Build history of the part. All positions in model axes, mm. Face numbers are marked on the shaded views. A direction names the side the tool comes from. Give positions to 0.01 mm unless a question says otherwise; leave off trailing zeros. Loops run counter-clockwise (first coordinate to the right, second up) from the corner with the lowest first, then second, coordinate; pieces in that order, holes last. Notation, with made-up numbers: (47, -2.5) - (60, -2.5) arc R24 ccw to (60, 34.5) - close; hole circle Ø3 at (-24, 25.5). An arc over 180 degrees is marked (long way). Return JSON: item names as keys, results as strings. Group by question number.
1) 3-axis set-ups, long thin cutter, end or side, ignore diameter. For the marked faces 5, 6 and 7: which of +Z, -Z, +X, -X, +Y, -Y reach the whole face in a straight line?
2) Slice it at B-B (z = 1.75). List the corners of the cut face in (x, y) (3 decimals), and give its area (3 significant figures).
3) Drill centre lines: probe 1 along Z at (x, y) = (10.5, 0.1) (1 decimal); probe 2 along X at (y, z) = (1.2, -9.5); probe 3 along X at (y, z) = (-0.05, -6). Where is each one in solid material? Low to high. Write a range as from..to.
4) Drop flat-ended pins along their axis: pin 1 (1 mm diameter, centred on x = 7.5, y = 0, fed in from +Z) (3 decimals); pin 2 (1 mm diameter, centred on x = -7, y = 1, fed in from -Z); pin 3 (1.5 mm diameter, centred on y = 0.5, z = 8.5, fed in from +X); pin 4 (3 mm diameter, centred on x = -5.5, z = -6, fed in from +Y) (3 decimals). Give the stop position or say it passes through.
5) Slice it at A-A (x = -0.5). List the corners of the cut face in (y, z) (3 decimals).
6) Mould opens along Z. For the marked faces 1, 2, 3 and 4 say: released by +Z, released by -Z, zero draft, split by the parting line, or undercut.
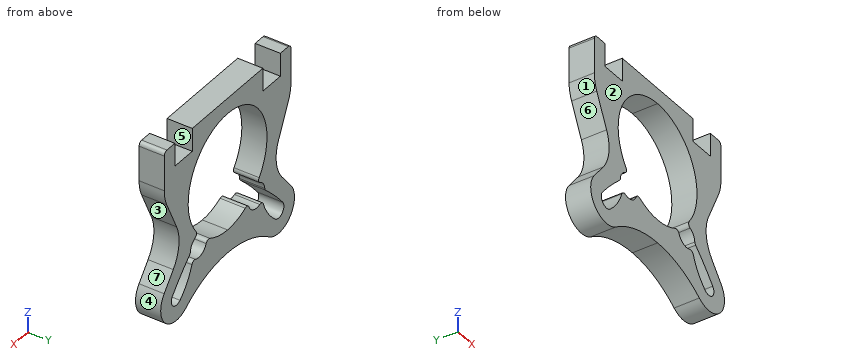
```python
from build123d import *
from build123d import SkipClean  # not in build123d's __all__

# Parameters (mm, degrees)
F2_DEPTH = 1.625
F3_R     = 0.5
F4_R     = 5


with BuildPart() as f2:
    # F1 (on Front) → F2 (new body, symmetric)
    with BuildSketch(Plane.XZ):
        with BuildLine():
            ThreePointArc((0, -6.875), (-2.0724417463, -6.5551971906), (-3.9520768911, -5.6255411515))
            ThreePointArc((-3.9520768911, -5.6255411515), (-4.8570002775, -7.1160909953), (-6.5757097792, -6.8217054979))
            ThreePointArc((-6.5757097792, -6.8217054979), (-7.4894639741, -8.9857797177), (-9.0066893746, -10.7791539234))
            ThreePointArc((-9.0066893746, -10.7791539234), (-10.3561219729, -10.7473840389), (-10.4445927673, -9.400479966))
            ThreePointArc((-10.4445927673, -9.400479966), (-8.8177667586, -7.5260240462), (-7.0479231089, -5.7859661986))
            ThreePointArc((-7.0479231089, -5.7859661986), (-6.6159518229, -4.6300438958), (-5.4766665535, -4.1559293139))
            ThreePointArc((-5.4766665535, -4.1559293139), (-6.837727437, 3.9011833784), (0, 8.375))
            Line((0, 8.375), (0, 10.375))
            Line((0, 10.375), (-6.6871520114, 10.375))
            Line((-6.6871520114, 10.375), (-6.6871520114, 7.375))
            Line((-6.6871520114, 7.375), (-9.9871520114, 7.375))
            Line((-9.9871520114, 7.375), (-9.9871520114, 10.375))
            Line((-9.9871520114, 10.375), (-11.9871520114, 10.375))
            Line((-11.9871520114, 10.375), (-11.9871520114, 4.2244328171))
            Line((-11.9871520114, 4.2244328171), (-8.5746230978, -3.0885299193))
            ThreePointArc((-8.5746230978, -3.0885299193), (-8.458137965, -3.3292198832), (-8.3348983214, -3.5665222959))
            Line((-8.3348983214, -3.5665222959), (-12.0057025921, -8.1503055323))
            ThreePointArc((-12.0057025921, -8.1503055323), (-11.8324993376, -12.098674705), (-7.8959026306, -12.4491384793))
            ThreePointArc((-7.8959026306, -12.4491384793), (-4.1524531082, -10.534781214), (0, -9.875))
            Line((0, -9.875), (0, -6.875))
        make_face()
    extrude(amount=F2_DEPTH, both=True)

    # F3
    f3_edges = [f2.edges().sort_by_distance(p)[0] for p in [
        (-3.952077, 0, -5.625541),
        (-7.047923, 0, -5.785966),
        (-11.987152, 0, 10.375),
        (-5.476667, 0, -4.155929),
        (-6.57571, 0, -6.821705),
    ]]
    fillet(f3_edges, radius=F3_R)

    # F4
    f4_edges = [f2.edges().sort_by_distance(p)[0] for p in [
        (-8.334898, 0, -3.566522),
        (-11.987152, 0, 4.224433),
    ]]
    fillet(f4_edges, radius=F4_R)

    # F5: F2 across plane


with BuildPart() as f2_1:
    add(f2.part, clean=False)
    with SkipClean():  # cleaning this boolean's faces spoils the solid; the shape is the same uncleaned
        add(f2.part.mirror(Plane.YZ), clean=False)


solid = f2_1.part
```
Results:
{
 "1": {"face 5": "+Z, +Y, -Y", "face 6": "-X, +Y, -Y", "face 7": "+X, +Y, -Y"},
 "2": {"outline": "(-10.832, -1.625) - (-7.415, -1.625) - (-7.415, 1.625) - (-10.832, 1.625) - close; (7.415, -1.625) - (10.832, -1.625) - (10.832, 1.625) - (7.415, 1.625) - close", "area": "22.2 mm2"},
 "3": {"probe 1": "-12.9..-10.6, -9.5..-6.3, 1..10.4", "probe 2": "-12.62..-10.51, -7.83..7.83, 10.51..12.62", "probe 3": "-10.28..-7.28, -3.82..-3.36, 3.36..3.82, 7.28..10.28"},
 "4": {"pin 1": "z = 7.375", "pin 2": "z = -12.17", "pin 3": "x = 11.99", "pin 4": "y = 1.625"},
 "5": {"outline": "(-1.625, -9.884) - (1.625, -9.884) - (1.625, -6.857) - (-1.625, -6.857) - close; (-1.625, 8.358) - (1.625, 8.358) - (1.625, 10.375) - (-1.625, 10.375) - close"},
 "6": {"face 1": "undercut", "face 2": "zero draft", "face 3": "undercut", "face 4": "split by the parting line"}
}
